Verification items for the finished model (mm, model axes). A direction names the side the tool comes from. Coordinates: 2 decimals unless noted, no trailing zeros. Write each loop counter-clockwise with the first axis right and the second up, starting at its lowest first coordinate (ties: lowest second). Pieces come first, ordered by that corner, then holes. Notation, with made-up numbers: (42, -20) -> (87, -20) arc R20 cw to (87, 16) -> close; hole circle Ø8 at (33.5, 85.5). An arc over 180 degrees is marked (long way). Answer in a Markdown table with one row per item.
Autodesk Inventor part; units mm, degrees
ref_plane "YZ Plane" through (0, 0, 0) normal (1, 0, 0) x (0, 1, 0)
ref_plane "XZ Plane" through (0, 0, 0) normal (0, 1, 0) x (-1, 0, 0)
ref_plane "XY Plane" through (0, 0, 0) normal (0, 0, 1) x (1, 0, 0)
sketch "スケッチ1" plane through (0, 0, 0) normal (0, 0, 1) x (1, 0, 0)
  line L0 (0, 0) -> (30, 0)
  line L1 (30, 0) -> (30, 20)
  line L2 (30, 20) -> (0, 20)
  line L3 (0, 20) -> (0, 0)
  dimension "d0" = 30
  dimension "d1" = 20
extrude "押し出し1" add sketch "スケッチ1" along normal blind 2
sketch "スケッチ2" plane through (0, 0, 2) normal (0, 0, 1) x (1, 0, 0)
  line L0 (0, 20) -> (0, 0)
  line L1 (0, 0) -> (30, 0)
  line L2 (30, 0) -> (30, 2)
  line L3 (30, 2) -> (0, 2)
  line L4 (0, 2) -> (0, 0)
  dimension "d4" = 2
extrude "押し出し2" add sketch "スケッチ2" along normal blind 300
fillet "フィレット1" radius 2 4 edges at (30, 20, 1) (0, 20, 1) (30, 1, 302) (0, 1, 302)
sketch "スケッチ3" plane through (0, 0, 0) normal (0, 0, -1) x (-1, 0, 0)
  line L0 (-28, 20) -> (-2, 20)
  line L1 (-15, 20) -> (-15, 0)
  line L2 (-2, 0) -> (-28, 0)
  point P0 (0, 0)
  point P1 (-24.7395, 16)
  point P2 (-5.2605, 16)
  point P3 (-24.7395, 6)
  point P4 (-5.2605, 6)
  dimension "d8" = 4
  dimension "d9" = 10
hole "穴1" at (24.7395, 16, 0) at (5.2605, 16, 0) at (24.7395, 6, 0) at (5.2605, 6, 0) direction (0, 0, 1) diameter 4.5 end through all
sketch "スケッチ4" plane through (0, 2, 2) normal (0, 1, 0) x (1, 0, 0)
  line L0 (2, -300) -> (28, -300)
  line L1 (15, -300) -> (15, 2) construction
  line L2 (28, 2) -> (2, 2)
  point P0 (0, 2)
  point P1 (15, -280)
  dimension "d17" = 20
hole "穴2" at (15, 2, 282) direction (0, -1, 0) diameter 7 end through all
sketch "スケッチ5" plane through (0, 2, 2) normal (0, 1, 0) x (1, 0, 0)
  line L0 (30, 0) -> (30, -298)
  line L1 (28, -8) -> (30, -8)
  line L2 (30, -8) -> (30, -260)
  line L3 (30, -260) -> (28, -260)
  line L4 (28, -260) -> (28, -8)
  line L5 (28, 2) -> (2, 2)
  line L6 (28, -300) -> (2, -300)
  line L7 (0, 0) -> (30, 0)
  line L8 (15, 0) -> (15, -300)
  line L9 (0, 0) -> (0, -298)
  line L10 (2, -8) -> (0, -8)
  line L11 (0, -8) -> (0, -260)
  line L12 (0, -260) -> (2, -260)
  line L13 (2, -260) -> (2, -8)
  point P0 (0, 2)
  dimension "d25" = 10
  dimension "d26" = 2
  dimension "d27" = 40
extrude "押し出し3" add sketch "スケッチ5" against normal blind 6
fillet "フィレット2" radius 1 4 edges at (29.4142, 2, 301.4142) (15, 2, 302) (0.5858, 2, 301.4142) (0, 2, 151)
properties part number "camera_stand" material "アルミニウム 6061"
1. Sectioned sample at A-A, the plane z = 282. Record the cut outline in (x, y), and give its area (3 significant figures).
Findings below:
| item | result |
|---|---|
| outline | (0, 0) -> (11.5, 0) -> (11.5, 2) -> (1, 2) arc R1 ccw to (0, 1) -> close; (18.5, 0) -> (30, 0) -> (30, 1) arc R1 ccw to (29, 2) -> (18.5, 2) -> close |
| area | 45.6 mm² |
2. Material ranges on probe 1 along X at (y, z) = (6, 0.85); probe 2 along X at (y, z) = (-2.5, 230.5); probe 3 along Z at (x, y) = (15, 1.1), recorded low to high. Write a range as from..to.
Findings below:
| item | result |
|---|---|
| probe 1 | x = 0..3.01, 7.51..22.49, 26.99..30 |
| probe 2 | x = 0..2, 28..30 |
| probe 3 | z = 0..278.5, 285.5..301.99 |
3. Sectioned sample at C-C, the plane z = 41. Record the cut outline in (x, y).
Findings below:
| item | result |
|---|---|
| outline | (0, -4) -> (2, -4) -> (2, 0) -> (28, 0) -> (28, -4) -> (30, -4) -> (30, 1) arc R1 ccw to (29, 2) -> (1, 2) arc R1 ccw to (0, 1) -> close |
4. Access from +Z, -Z, +X, -X, +Y, -Y to the whole of each face (thin tool, end or side, straight path). Record for faces 4 (the face through (15, 10, 0)), 5 (the face through (15, 2, 149)).
Findings below:
| item | result |
|---|---|
| face 4 | -Z, +X, -X, +Y, -Y |
| face 5 | +Z, +X, -X, +Y |
5. Release check for a two-part mould opening along Z. For faces 1 (the face through (0, -1, 138)), 2 (the face through (15, 11, 2)), 3 (the face through (13.95, 0.99, 285.34)) record: released by +Z, released by -Z, zero draft, split by the parting line, or undercut.
Findings below:
| item | result |
|---|---|
| face 1 | zero draft |
| face 2 | released by +Z |
| face 3 | undercut |
6. Go/stop test with flat-tipped pins: pin 1 (12 mm diameter, centred on y = 12.5, z = 194, fed in from -X); pin 2 (0.6 mm diameter, centred on x = 29, y = -2.5, fed in from +Z); pin 3 (9.5 mm diameter, centred on x = 17, y = 14, fed in from +Z); pin 4 (0.6 mm diameter, centred on x = 1.5, y = -1.5, fed in from -Z). Record where each tip stops, or that it passes through.
Findings below:
| item | result |
|---|---|
| pin 1 | passes through |
| pin 2 | stops at z = 262 |
| pin 3 | stops at z = 2 |
| pin 4 | stops at z = 10 |
7. Sectioned sample at B-B, the plane x = 15. Record the cut outline in (y, z).
Findings below:
| item | result |
|---|---|
| outline | (0, 0) -> (20, 0) -> (20, 2) -> (2, 2) -> (2, 278.5) -> (0, 278.5) -> close; (0, 285.5) -> (2, 285.5) -> (2, 301) arc R1 ccw to (1, 302) -> (0, 302) -> close |
